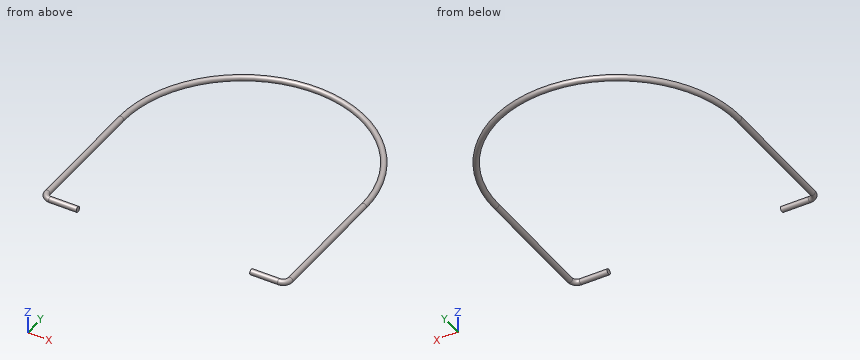
```python
from build123d import *

# Parameters (mm, degrees)
SKETCH2_R = 1.5875


with BuildPart() as part:
    # Sweep1: sweep along a path in Sketch1
    with BuildLine(Plane.XY) as sweep1_path:
        Line((0, 0), (-16, 0))
        ThreePointArc((-16, 0), (-18.828427125, 1.171572875), (-20, 4))
        Line((-20, 4), (-20, 75))
        ThreePointArc((-20, 75), (50, 145), (120, 75))
        Line((120, 75), (120, 4))
        ThreePointArc((120, 4), (118.828427125, 1.171572875), (116, 0))
        Line((116, 0), (100, 0))
    # Sketch2 → Sweep1 (sweep)
    with BuildSketch(Plane(origin=(0, 0, 0), x_dir=(0, 0, -1), z_dir=(1, 0, 0))):
        Circle(SKETCH2_R)
    sweep(path=sweep1_path.line)


solid = part.part
```
Work out the finished part from the listing and answer in its coordinate system (mm). Coordinates: 2 decimals unless noted, no trailing zeros. Write each loop counter-clockwise with the first axis right and the second up, starting at its lowest first coordinate (ties: lowest second). Pieces come first, ordered by that corner, then holes.
Q1. Each of these flat-tipped pins is pushed along its axis until it touches: pin 1 Ø1.6 at (y, z) = (-0.5, -0.5) entering from +X; pin 2 Ø1.5 at (y, z) = (103, -0.5) entering from +X. Where does it stop, or does it pass through?
Q2. A cutting plane is placed at C-C, the plane x = 50. Give the vertices of the cut face in (y, z) (1 decimal), then the cut area to 3 significant figures.
Q3. A cutting plane is placed at B-B, the plane y = 46. Give the vertices of the cut face in (x, z) (1 decimal).
Q4. A cutting plane is placed at A-A, the plane z = 0. Give the vertices of the cut face in (x, y) (1 decimal).
Q5. Find the intervals of material crossed by line 1 (X direction, y = 67, z = 0.1); line 2 (X direction, y = 82, z = 1.1); line 3 (Y direction, x = -9.5, z = -1.2), in increasing order.
Findings below:
1. pin 1: stops at x = 120.13
1. pin 2: stops at x = 116.16
2. outline: circle Ø3.2 at (145, 0)
2. area: 7.92 mm2
3. outline: circle Ø3.2 at (-20, 0); circle Ø3.2 at (120, 0)
4. outline: (-21.6, 4) arc R5.6 ccw to (-16, -1.6) - (0, -1.6) - (0, 1.6) - (-16, 1.6) arc R2.4 cw to (-18.4, 4) - (-18.4, 75) arc R68.4 cw to (118.4, 75) - (118.4, 4) arc R2.4 cw to (116, 1.6) - (100, 1.6) - (100, -1.6) - (116, -1.6) arc R5.6 ccw to (121.6, 4) - (121.6, 75) arc R71.6 ccw to (-21.6, 75) - close
5. line 1: x = -21.58 to -18.42, 118.42 to 121.58
5. line 2: x = -20.8 to -18.5, 118.5 to 120.8
5. line 3: y = -1.04 to 1.04, 109.86 to 113.81
